```python
from build123d import *

# Parameters (mm, degrees)
SKETCH1_W           = 490
SKETCH1_H           = 98.65
BOSS_EXTRUDE1_DEPTH = 6
SKETCH2_W           = 6
SKETCH2_H           = 24
SKETCH2_W_2         = 333.333333334
SKETCH2_H_2         = 6
CUT_EXTRUDE1_DEPTH  = 500.867805024


with BuildPart() as part:
    # Sketch1 → Boss-Extrude1 (new body)
    with BuildSketch(Plane.XY):
        with Locations((245, 49.325)):
            Rectangle(SKETCH1_W, SKETCH1_H)
    extrude(amount=BOSS_EXTRUDE1_DEPTH)

    # Sketch2 → Cut-Extrude1 (cut, through all)
    with BuildSketch(Plane.XY.offset(6)):
        with Locations((487, 86.65)):
            Rectangle(SKETCH2_W, SKETCH2_H)
        with Locations((487, 12)):
            Rectangle(SKETCH2_W, SKETCH2_H)
        with Locations((3, 12)):
            Rectangle(SKETCH2_W, SKETCH2_H)
        with Locations((3, 86.65)):
            Rectangle(SKETCH2_W, SKETCH2_H)
        with Locations((245, 95.65)):
            Rectangle(SKETCH2_W_2, SKETCH2_H_2)
        with Locations((245, 3)):
            Rectangle(SKETCH2_W_2, SKETCH2_H_2)
    extrude(amount=-CUT_EXTRUDE1_DEPTH, mode=Mode.SUBTRACT)


solid = part.part
```
Model file for the job. Use its own axes, mm. Give positions to 0.01 mm unless a question says otherwise; leave off trailing zeros. Order: outer loops, then holes, each group sorted by start corner. A loop starts at its lowest first (then second) coordinate and runs counter-clockwise, first axis right, second up.
1) Pin check, flat tips, straight feed: pin 1 (1.8 mm diameter, centred on y = 96, z = 2.5, fed in from -X); pin 2 (1.5 mm diameter, centred on y = 83, z = 4.5, fed in from +X); pin 3 (1.8 mm diameter, centred on x = 325, z = 3.5, fed in from -Y). Stop position of each tip, or through.
2) Saw through at B-B, the plane y = 83. Write the cut outline in (x, z), then the cut area to 3 significant figures.
3) Wall check: probe 1 along X at (y, z) = (94, 1.75); probe 2 along X at (y, z) = (16, 1.7); probe 3 along Y at (x, z) = (320, 4). Give the ranges that are in metal, low to high.
4) Saw through at A-A, the plane z = 4.4. Write the cut outline in (x, y).
5) Saw through at C-C, the plane x = 204.5. Write the cut outline in (y, z), then the cut area to 3 significant figures.
Computed:
1. pin 1: stops at x = 6
1. pin 2: stops at x = 484
1. pin 3: stops at y = 6
2. outline: (6, 0) - (484, 0) - (484, 6) - (6, 6) - close
2. area: 2,870 mm2
3. probe 1: x = 6 to 78.33, 411.67 to 484
3. probe 2: x = 6 to 484
3. probe 3: y = 6 to 92.65
4. outline: (0, 24) - (6, 24) - (6, 0) - (78.33, 0) - (78.33, 6) - (411.67, 6) - (411.67, 0) - (484, 0) - (484, 24) - (490, 24) - (490, 74.65) - (484, 74.65) - (484, 98.65) - (411.67, 98.65) - (411.67, 92.65) - (78.33, 92.65) - (78.33, 98.65) - (6, 98.65) - (6, 74.65) - (0, 74.65) - close
5. outline: (6, 0) - (92.65, 0) - (92.65, 6) - (6, 6) - close
5. area: 520 mm2
